Print and shaded views of the part. All mm, measured from the part's lowest x, y and z. Give positions to 0.01 mm unless a question says otherwise; leave off trailing zeros. Write each loop counter-clockwise with the first axis right and the second up, starting at its lowest first coordinate (ties: lowest second). Pieces come first, ordered by that corner, then holes. Notation, with made-up numbers: (-17, -15.5) -> (14, -15.5) arc R30 cw to (14, 12.5) -> close; hole circle Ø6 at (18.25, -2.75). An arc over 180 degrees is marked (long way). Put each result on its own line as item: value.
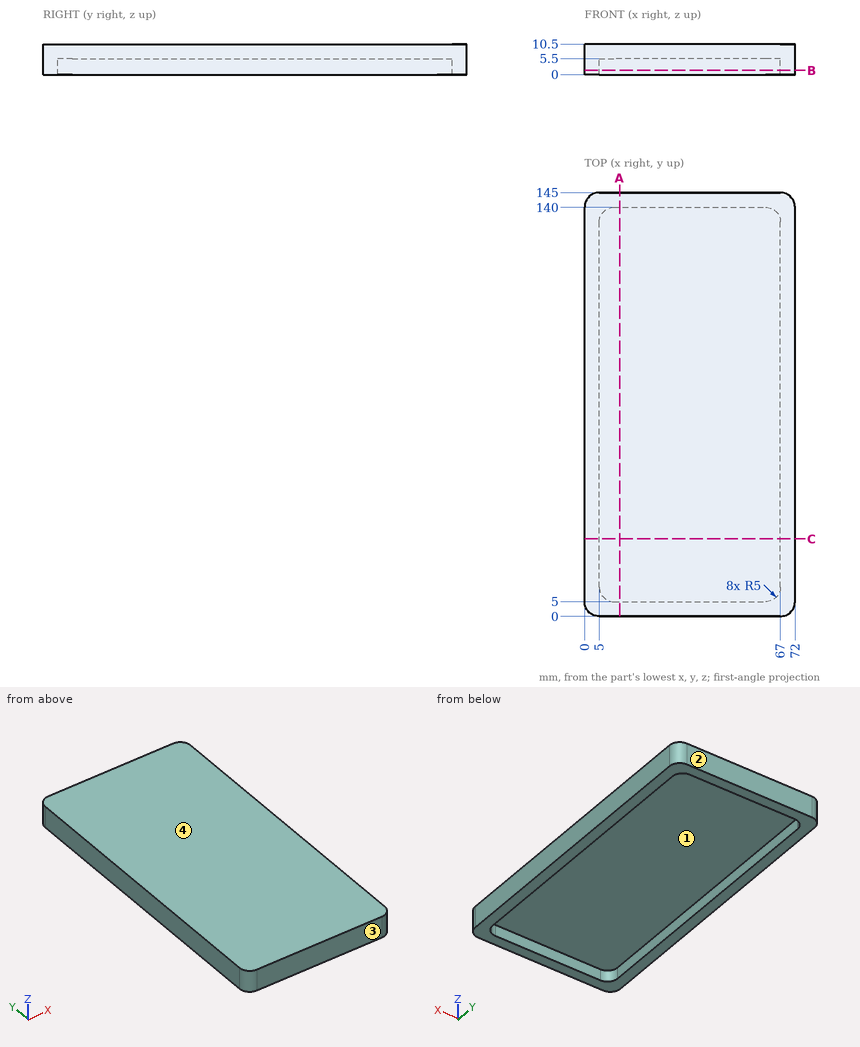
1) Slice it at B-B (z = 1.5). Write the cut outline in (x, y).
Filled sheet:
outline: (0, 5) arc R5 ccw to (5, 0) -> (67, 0) arc R5 ccw to (72, 5) -> (72, 140) arc R5 ccw to (67, 145) -> (5, 145) arc R5 ccw to (0, 140) -> close; hole (5, 10) arc R5 ccw to (10, 5) -> (62, 5) arc R5 ccw to (67, 10) -> (67, 135) arc R5 ccw to (62, 140) -> (10, 140) arc R5 ccw to (5, 135) -> close
2) Pin check, flat tip, straight feed: pin 1 (1.5 mm diameter, centred on x = 31, y = 39, fed in from -Z). Stop position of the tip, or through.
Filled sheet:
pin 1: z = 5.5
3) Wall check: L1, parallel to X at y = 134.5, z = 4.75; L2, parallel to Y at x = 42.5, z = 3.75; L3, parallel to Z at x = 24, y = 110. Give the ranges that are in metal, low to high.
Filled sheet:
L1: 0 to 5, 67 to 72
L2: 0 to 5, 140 to 145
L3: 5.5 to 10.5
4) Pull direction Y, two halves, no side cores. Call the marked faces 1, 2, 3 and 4: released by +Y, released by -Y, zero draft, split by the parting line, or undercut.
Filled sheet:
face 1: undercut
face 2: released by +Y
face 3: released by -Y
face 4: zero draft
5) Slice it at C-C (y = 26.5). Write the cut outline in (x, z), plus the area to 3 significant figures.
Filled sheet:
outline: (0, 0) -> (5, 0) -> (5, 5.5) -> (67, 5.5) -> (67, 0) -> (72, 0) -> (72, 10.5) -> (0, 10.5) -> close
area: 415 mm2
6) Slice it at A-A (x = 12). Write the cut outline in (y, z), plus the area to 3 significant figures.
Filled sheet:
outline: (0, 0) -> (5, 0) -> (5, 5.5) -> (140, 5.5) -> (140, 0) -> (145, 0) -> (145, 10.5) -> (0, 10.5) -> close
area: 780 mm2
